Build history of the part. All positions in model axes, mm. A direction names the side the tool comes from. Round coordinates to 2 decimals unless told otherwise and drop trailing zeros. Write each loop counter-clockwise with the first axis right and the second up, starting at its lowest first coordinate (ties: lowest second). Pieces come first, ordered by that corner, then holes. Notation, with made-up numbers: (-18, 55.25) -> (-1, 55.25) arc R24 cw to (-1, 93.25) -> close; hole circle Ø11 at (-4, 88.25). An arc over 180 degrees is marked (long way). Answer in a Markdown table with one row per item.
```python
from build123d import *

# Parameters (mm, degrees)
CUT_EXTRUDE1_REACH                  = 31.419
CUT_EXTRUDE1_END_RADIUS             = 2.95
SKETCH2_R                           = 1.5
CUT_EXTRUDE1_DIRECTION_2_REACH      = 31.419
CUT_EXTRUDE1_DIRECTION_2_END_RADIUS = 2.95
FILLET1_R                           = 0.1


with BuildPart() as part:
    # Sketch1 → Revolve1 (revolve)
    with BuildSketch(Plane(origin=(0, 0, 0), x_dir=(1, 0, 0), z_dir=(0, 1, 0)), mode=Mode.PRIVATE) as revolve1_sk:
        Polygon((-29, 0), (0, 0), (0, 3.5), (-1, 3.5), (-1, 2.95), (-13, 2.95), (-13, 2.45), (-22.5, 2.45), (-22.5, 2), (-29, 2), align=None)
    revolve(revolve1_sk.sketch.rotate(Axis((-33.923612536, 0, 0), (1, 0, 0)), 180), axis=Axis((-33.923612536, 0, 0), (1, 0, 0)))

    # Cut-Extrude1: up to this cylinder (the profile starts inside it)
    cut_extrude1_end = Plane(origin=(-7, 0, 0), z_dir=(-1, 0, 0)) * Cylinder(CUT_EXTRUDE1_END_RADIUS, 69.738, mode=Mode.PRIVATE)
    # Sketch2 → Cut-Extrude1 (cut, up to the surface)
    with BuildSketch(Plane.XY, mode=Mode.PRIVATE) as cut_extrude1_sk1:
        with Locations((-7, 0)):
            Circle(SKETCH2_R)
    cut_extrude1_tool1 = extrude(cut_extrude1_sk1.sketch, amount=-CUT_EXTRUDE1_REACH, mode=Mode.PRIVATE) & cut_extrude1_end
    add(cut_extrude1_tool1.solids().sort_by_distance((-7, 0, 0))[0], mode=Mode.SUBTRACT)

    # Cut-Extrude1 direction 2: up to this cylinder (the profile starts inside it)
    cut_extrude1_direction_2_end = Plane(origin=(-7, 0, 0), z_dir=(-1, 0, 0)) * Cylinder(CUT_EXTRUDE1_DIRECTION_2_END_RADIUS, 69.738, mode=Mode.PRIVATE)
    # Sketch2 → Cut-Extrude1 direction 2 (cut, up to the surface)
    with BuildSketch(Plane.XY, mode=Mode.PRIVATE) as cut_extrude1_direction_2_sk1:
        with Locations((-7, 0)):
            Circle(SKETCH2_R)
    cut_extrude1_direction_2_tool1 = extrude(cut_extrude1_direction_2_sk1.sketch, amount=CUT_EXTRUDE1_DIRECTION_2_REACH, mode=Mode.PRIVATE) & cut_extrude1_direction_2_end
    add(cut_extrude1_direction_2_tool1.solids().sort_by_distance((-7, 0, 0))[0], mode=Mode.SUBTRACT)

    # Fillet1
    fillet1_edges = [part.edges().sort_by_distance(p)[0] for p in [
        (0, 0, -3.5),
    ]]
    fillet(fillet1_edges, radius=FILLET1_R)


solid = part.part
```
Q1. Saw through at A-A on y = 0. Write the cut outline in (x, z).
A:
| item | result |
|---|---|
| outline | (-29, -2) -> (-22.5, -2) -> (-22.5, -2.45) -> (-13, -2.45) -> (-13, -2.95) -> (-8.5, -2.95) -> (-8.5, 2.95) -> (-13, 2.95) -> (-13, 2.45) -> (-22.5, 2.45) -> (-22.5, 2) -> (-29, 2) -> close; (-5.5, -2.95) -> (-1, -2.95) -> (-1, -3.5) -> (-0.1, -3.5) arc R0.1 ccw to (0, -3.4) -> (0, 3.4) arc R0.1 ccw to (-0.1, 3.5) -> (-1, 3.5) -> (-1, 2.95) -> (-5.5, 2.95) -> close |
Q2. Saw through at B-B on z = 0. Write the cut outline in (x, y).
A:
| item | result |
|---|---|
| outline | (-29, -2) -> (-22.5, -2) -> (-22.5, -2.45) -> (-13, -2.45) -> (-13, -2.95) -> (-1, -2.95) -> (-1, -3.5) -> (-0.1, -3.5) arc R0.1 ccw to (0, -3.4) -> (0, 3.4) arc R0.1 ccw to (-0.1, 3.5) -> (-1, 3.5) -> (-1, 2.95) -> (-13, 2.95) -> (-13, 2.45) -> (-22.5, 2.45) -> (-22.5, 2) -> (-29, 2) -> close; hole circle Ø3 at (-7, 0) |
Q3. Wall check: line 1 (X direction, y = 0, z = -0.95); line 2 (X direction, y = -1.25, z = -1); line 3 (Y direction, x = -7, z = 0.2). Give the ranges that are in metal, low to high. Write a range as [from, to].
A:
| item | result |
|---|---|
| line 1 | [-29, -8.5], [-5.5, 0] |
| line 2 | [-29, -7.83], [-6.17, 0] |
| line 3 | [-2.94, -1.5], [1.5, 2.94] |
Q4. Drop flat-ended pins along their axis: P1, Ø3, axis at x = -11.5, y = -2.5, coming from the -Z side; P2, Ø1, axis at y = -0.5, z = -2.5, coming from the -X side; P3, Ø4, axis at x = -10.5, y = -1.5, coming from the +Z side. Give the stop position or say it passes through.
A:
| item | result |
|---|---|
| P1 | z = -2.78 |
| P2 | x = -22.5 |
| P3 | z = 2.95 |
Q5. Saw through at D-D on x = -3.5. Write the cut outline in (y, z).
A:
| item | result |
|---|---|
| outline | circle Ø5.9 at (0, 0) |
Q6. Which spindle directions (+Z, -Z, +X, -X, +Y, -Y) get a long thin tool onto all of the face, cutting with end or side? Do faces 1 (the cylindrical face through (-0.556, 1.341, 3.233)), 2 (the flat face through (-22.5, 2, -1)). Say none if no direction does.
A:
| item | result |
|---|---|
| face 1 | +X, -X |
| face 2 | -X |
Q7. Saw through at C-C on x = -27. Write the cut outline in (y, z).
A:
| item | result |
|---|---|
| outline | circle Ø4 at (0, 0) |
Q8. Two-plate mould, pull along X, no slides. Class faces 3 (the flat face through (0, 0, 0)), 4 (the flat face through (-1, 1, -3)), 5 (the cylindrical face through (-6.194, 1.265, -0.041)): released by +X, released by -X, zero draft, split by the parting line, or undercut.
A:
| item | result |
|---|---|
| face 3 | released by +X |
| face 4 | released by -X |
| face 5 | undercut |
